Input: part model. Units: mm. Frame: model coordinates. Give positions to 0.01 mm unless a question says otherwise; leave off trailing zeros. Write each loop counter-clockwise with the first axis right and the second up, starting at its lowest first coordinate (ties: lowest second). Pieces come first, ordered by that corner, then holes. Notation, with made-up numbers: (-32.75, 67) - (-8.75, 67) arc R32 ccw to (-8.75, 99) - close; hole circle Ø6 at (2.25, 74.5). An arc over 180 degrees is marked (long way). Use a Markdown table: item, result. Add a question column.
1. Section query C-C, the plane x = 0. Return loops of the section in (y, z).
2. Section query B-B, the plane y = 4.75. Count the separate pieces of the cut face and the enclosed holes in it, plus the area to 3 significant figures.
3. Material intervals for probe 1 along X at (y, z) = (11, 21); probe 2 along Z at (x, y) = (-12.5, 11.25); probe 3 along X at (y, z) = (4.75, 21), sorted ascending.
4. Pin query (flat end, axial travel): pin 1 (3 mm diameter, centred on x = -12.5, z = 39, fed in from +Y); pin 2 (6 mm diameter, centred on x = 11.5, z = -22, fed in from -Y); pin 3 (4 mm diameter, centred on x = -5.5, z = 48, fed in from +Y). Return the tip coordinate at first contact, or that it passes through.
5. Section query A-A, the plane z = -39. Return loops of the section in (x, y).
Autodesk Fusion 360 part; units mm, degrees
sketch "Board" plane through (0, 0, 0) normal (0, 1, 0) x (1, 0, 0)
  line L0 (-25, -45) -> (-25, -50)
  circle A0 centre (12.5, -39) radius 6
  line L1 (-25, -50) -> (25, -50)
  circle A1 centre (12.5, -21) radius 2.5
  circle A2 centre (12.5, 21) radius 2.5
  line L2 (-25, 50) -> (25, 50)
  circle A3 centre (0, 30) radius 1.5
  line L3 (-25, 45) -> (-25, 50)
  circle A4 centre (12.5, 39) radius 6
  circle A5 centre (-12.5, 21) radius 2.5
  circle A6 centre (12.5, 21) radius 6
  line L4 (25, 50) -> (25, 45)
  circle A7 centre (12.5, -21) radius 6
  line L5 (-25, 50) -> (25, 50)
  circle A8 centre (-12.5, 21) radius 6
  circle A9 centre (-12.5, -21) radius 2.5
  line L6 (25, 50) -> (-25, 50)
  circle A10 centre (12.5, 39) radius 2.5
  circle A11 centre (-12.5, 39) radius 6
  circle A12 centre (-12.5, 39) radius 2.5
  line L7 (25, -45) -> (-25, -45)
  line L8 (25, -50) -> (-25, -50)
  circle A13 centre (12.5, -39) radius 2.5
  circle A14 centre (-12.5, -39) radius 6
  circle A15 centre (0, -30) radius 1.5
  circle A16 centre (-12.5, -39) radius 2.5
  line L9 (25, -50) -> (25, -45)
  line L10 (25, 50) -> (25, -50)
  line L11 (25, 45) -> (-25, 45)
  line L12 (-25, -50) -> (-25, 50)
  circle A17 centre (0, 0) radius 1.5
  circle A18 centre (-12.5, -21) radius 6
  dimension "d23" = 100
  dimension "d24" = 5
  dimension "d25" = 5
  dimension "d26" = 5
  dimension "d27" = 5
  dimension "d28" = 5
  dimension "d29" = 5
  dimension "d30" = 5
  dimension "d31" = 5
  dimension "d32" = 3
  dimension "d33" = 3
  dimension "d34" = 3
  dimension "d35" = 12
  dimension "d36" = 12
  dimension "d37" = 12
  dimension "d38" = 12
  dimension "d39" = 12
  dimension "d40" = 12
  dimension "d41" = 12
  dimension "d42" = 12
  dimension "d43" = 5
  dimension "d44" = 5
extrude "Extrude1" add sketch "Board" along normal blind 13 contours L0 L1 L7 L8 L9 L10 L12 | L2 L3 L4 L5 L6 L10 L11 L12 makes body 1 at (8.3333, 4.3333, 45) makes body 2 at (-8.3333, 4.3333, -50)
extrude "Extrude2" add sketch "Board" along normal blind 18 contours A14 | A0 | A4 | A11 | L7 L10 L11 L12 | A3 | A6 | A7 | A8 | A15 | A17 | A18 bodies 1 2
extrude "Extrude3" cut sketch "Board" along normal blind 7 contours A14 | A0 | A4 | A11 | A6 | A7 | A8 | A18 bodies 1
extrude "Extrude4" cut sketch "Board" along normal blind 7 contours A3 | A15 | A17 bodies 1
chamfer "Chamfer1" distance 2 angle 45 2 edges at (25, 0, 0) (-25, 0, 0) on bodies 1
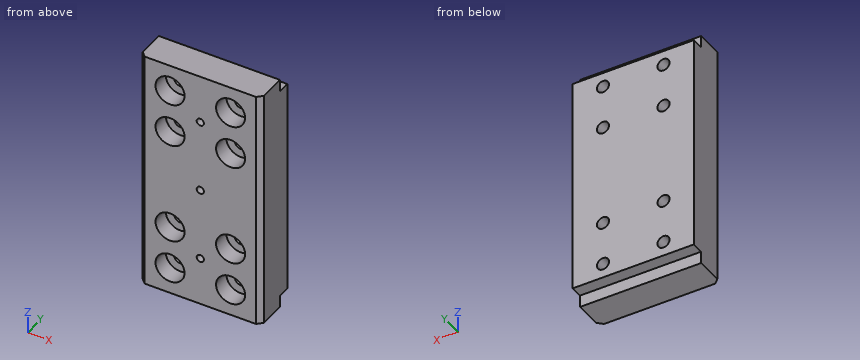
Result sheet:
| question | item | result |
|---|---|---|
| 1 | outline | (0, -50) - (13, -50) - (13, -45) - (18, -45) - (18, 45) - (13, 45) - (13, 50) - (0, 50) - (0, 31.5) - (7, 31.5) - (7, 28.5) - (0, 28.5) - (0, 1.5) - (7, 1.5) - (7, -1.5) - (0, -1.5) - (0, -28.5) - (7, -28.5) - (7, -31.5) - (0, -31.5) - close |
| 2 | separate pieces | 1 |
| 2 | enclosed holes | 11 |
| 2 | area | 4,070 mm² |
| 3 | probe 1 | x = -25 to -15, -10 to 10, 15 to 25 |
| 3 | probe 2 | z = -50 to -41.5, -36.5 to -23.5, -18.5 to 18.5, 23.5 to 36.5, 41.5 to 50 |
| 3 | probe 3 | x = -25 to -18.5, -6.5 to 6.5, 18.5 to 25 |
| 4 | pin 1 | passes through |
| 4 | pin 2 | stops at y = 7 |
| 4 | pin 3 | stops at y = 13 |
| 5 | outline | (-25, 2) - (-23, 0) - (-18.5, 0) - (-18.5, 7) - (-15, 7) - (-15, 18) - (-25, 18) - close; (-10, 7) - (-6.5, 7) - (-6.5, 0) - (6.5, 0) - (6.5, 7) - (10, 7) - (10, 18) - (-10, 18) - close; (15, 7) - (18.5, 7) - (18.5, 0) - (23, 0) - (25, 2) - (25, 18) - (15, 18) - close |
